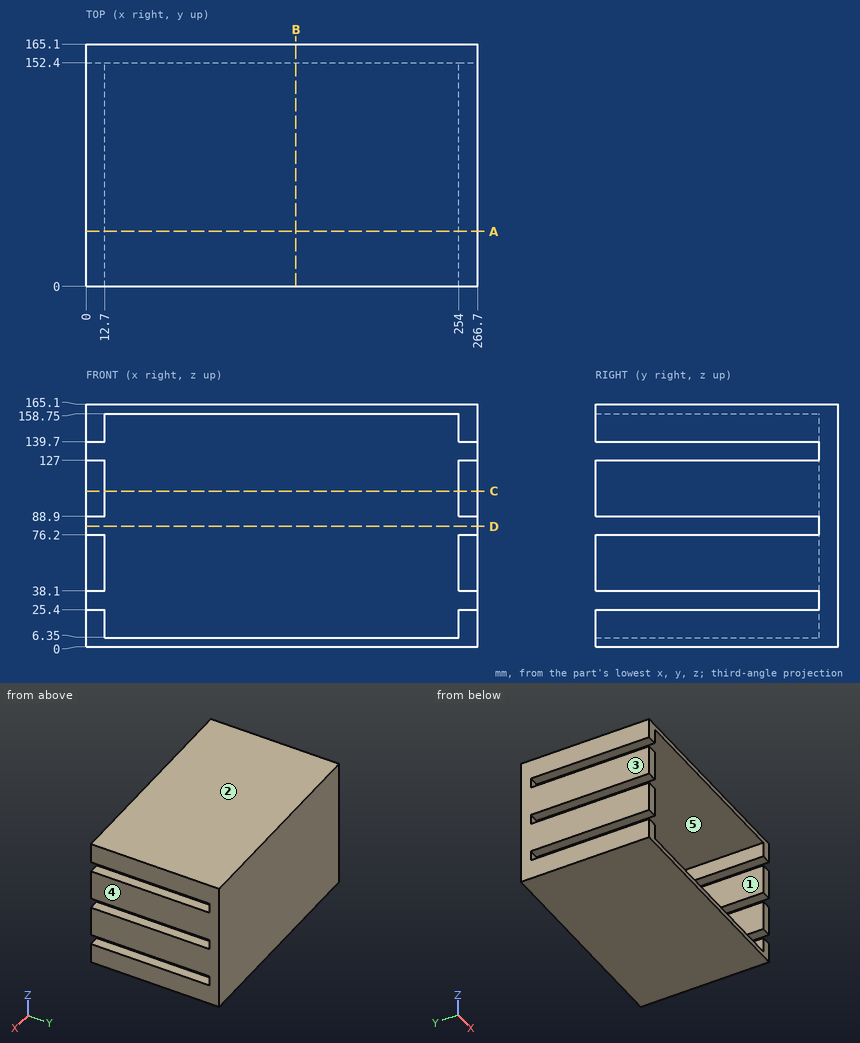
Answer from the drawing. Dimensions are ordinates in mm from the lowest x, y and z of the part. A direction names the side the tool comes from. Give positions to 0.01 mm unless a question says otherwise; leave off trailing zeros. Order: outer loops, then holes, each group sorted by start corner. A loop starts at its lowest first (then second) coordinate and runs counter-clockwise, first axis right, second up. Notation, with made-up numbers: (-39.5, 59) - (9.5, 59) arc R25 cw to (9.5, 75) - close; hole circle Ø9 at (15, 57.5). An arc over 180 degrees is marked (long way). One line per item, written item: value. Start each with the question number.
1. Consider line 1 (Z direction, x = 52.5, y = 52); line 2 (X direction, y = 86, z = 114); line 3 (Y direction, x = 71.5, z = 134). Determine where each line is inside the solid, lowest interval first.
2. Section A-A, the plane y = 37.5 is taken. Count the separate pieces of the cut face and the enclosed holes in it, then the cut area to 3 significant figures.
3. Section C-C, the plane z = 106 is taken. Write down the section's boundary in (x, y).
4. Section D-D, the plane z = 82 is taken. Write down the section's boundary in (x, y).
5. For a pull along X with two mould halves and no side action, classify the marked faces 3, 4 and 5 as released by +X, released by -X, zero draft, split by the parting line, or undercut.
6. Section B-B, the plane x = 143 is taken. Write down the section's boundary in (y, z), then the cut area to 3 significant figures.
7. Which of the six approach directions +Z, -Z, +X, -X, +Y, -Y give full straight-line access (tool end or side, diameter ignored) to the marked faces 1 and 2?
8. Each of these flat-tipped pins is pushed along its axis until it touches: pin 1 Ø10 at (x, y) = (8.5, 39) entering from -Z; pin 2 Ø8 at (y, z) = (87.5, 81.5) entering from -X; pin 3 Ø10 at (x, z) = (140.5, 90) entering from -Y. Where does it stop, or does it pass through?
Filled sheet:
1. line 1: 0 to 6.35, 158.75 to 165.1
1. line 2: 0 to 12.7, 254 to 266.7
1. line 3: 152.4 to 165.1
2. separate pieces: 6
2. enclosed holes: 0
2. area: 6,290 mm²
3. outline: (0, 0) - (12.7, 0) - (12.7, 152.4) - (254, 152.4) - (254, 0) - (266.7, 0) - (266.7, 165.1) - (0, 165.1) - close
4. outline: (0, 152.4) - (266.7, 152.4) - (266.7, 165.1) - (0, 165.1) - close
5. face 3: released by -X
5. face 4: released by +X
5. face 5: undercut
6. outline: (0, 0) - (165.1, 0) - (165.1, 165.1) - (0, 165.1) - (0, 158.75) - (152.4, 158.75) - (152.4, 6.35) - (0, 6.35) - close
6. area: 4,030 mm²
7. face 1: -Y
7. face 2: +Z, +X, -X, +Y, -Y
8. pin 1: z = 0
8. pin 2: through
8. pin 3: y = 152.4
